```python
from build123d import *

# Parameters (mm, degrees)
CUT_EXTRUDE1_REACH                              = 51.117
CBORE_FOR_M4_SOCKET_HEAD_CAP_SCREW1_D           = 4.5
CBORE_FOR_M4_SOCKET_HEAD_CAP_SCREW1_CBORE_D     = 8
CBORE_FOR_M4_SOCKET_HEAD_CAP_SCREW1_CBORE_DEPTH = 4.4
CHAMFER1_SIZE                                   = 1
CHAMFER2_SIZE                                   = 0.3


with BuildPart() as part:
    # Sketch1 → Revolve1 (revolve)
    with BuildSketch(Plane.XY, mode=Mode.PRIVATE) as revolve1_sk:
        Polygon((-21, 0), (-21, 16.5), (0, 16.5), (0, 27.5), (9, 27.5), (9, 16.5), (28, 16.5), (28, 0), align=None)
    revolve(revolve1_sk.sketch.rotate(Axis((-30.202765387, 0, 0), (1, 0, 0)), 90), axis=Axis((-30.202765387, 0, 0), (1, 0, 0)))

    # Sketch2 → Cut-Revolve1 (revolve, cut)
    with BuildSketch(Plane.XY, mode=Mode.PRIVATE) as cut_revolve1_sk:
        Polygon((-21, 0), (-21, 13), (-5, 13), (-5, 11), (20, 11), (20, 13), (28, 13), (28, 0), align=None)
    revolve(cut_revolve1_sk.sketch.rotate(Axis((-25.491403617, 0, 0), (1, 0, 0)), 90), axis=Axis((-25.491403617, 0, 0), (1, 0, 0)), mode=Mode.SUBTRACT)

    # Sketch5 → Cut-Extrude1 (cut, up to next)
    with BuildSketch(Plane(origin=(9, 0, 0), x_dir=(0, 0, -1), z_dir=(1, 0, 0)), mode=Mode.PRIVATE) as cut_extrude1_sk1:
        with BuildLine():
            Line((18.5, 20.346989949), (18.5, -20.346989949))
            ThreePointArc((18.5, -20.346989949), (27.5, 0), (18.5, 20.346989949))
        make_face()
    cut_extrude1_tool1 = extrude(cut_extrude1_sk1.sketch, amount=-CUT_EXTRUDE1_REACH, mode=Mode.PRIVATE) & part.part
    add(cut_extrude1_tool1.solids().sort_by_distance((9, 0, -22.155812))[0], mode=Mode.SUBTRACT)

    # CBORE for M4 Socket Head Cap Screw1 (through all)
    with Locations(Plane(origin=(9, 0, 0), x_dir=(0, 0, -1), z_dir=(1, 0, 0))):
        with Locations((-13.25, 18), (13.25, 18), (13.25, -18), (-13.25, -18)):
            CounterBoreHole(CBORE_FOR_M4_SOCKET_HEAD_CAP_SCREW1_D / 2, CBORE_FOR_M4_SOCKET_HEAD_CAP_SCREW1_CBORE_D / 2, CBORE_FOR_M4_SOCKET_HEAD_CAP_SCREW1_CBORE_DEPTH)

    # Chamfer1
    chamfer1_edges = [part.edges().sort_by_distance(p)[0] for p in [
        (-21, 0, -16.5),
    ]]
    chamfer(chamfer1_edges, length=CHAMFER1_SIZE)

    # Chamfer2
    chamfer2_edges = [part.edges().sort_by_distance(p)[0] for p in [
        (28, 0, -16.5),
    ]]
    chamfer(chamfer2_edges, length=CHAMFER2_SIZE)


solid = part.part
```
Geometry: final body of the model. Coordinates: model frame, mm. A direction names the side the tool comes from. Round coordinates to 2 decimals unless told otherwise and drop trailing zeros. Write each loop counter-clockwise with the first axis right and the second up, starting at its lowest first coordinate (ties: lowest second). Pieces come first, ordered by that corner, then holes. Notation, with made-up numbers: M 81,-12.5 L 111,-12.5 A22 cw 111,2.5 Z; hole C -27.5,62 d9. An arc over 180 degrees is marked long. Answer in a Markdown table with one row per item. Add a question column.
(1) Ray query, L1, parallel to Y at x = 2.95, z = 13.25; L2, parallel to Y at x = 3, z = -12; L3, parallel to X at y = 19.5, z = -16. Return the intervals inside material, ascending.
(2) Contact query for flat-ended pins moving along their axis: pin 1 (12 mm diameter, centred on x = 17.5, z = 12.5, fed in from -Y); pin 2 (5 mm diameter, centred on x = 15.5, y = 10, fed in from +Z); pin 3 (12 mm diameter, centred on x = -7.5, z = -1, fed in from -Y). Output: stop coordinate, or through.
(3) Cut plane C-C, the plane y = 0. Return the cut outline in (x, z), then the cut area to 3 significant figures.
(4) Draft query along Z for faces 1 (the face through (28, -13.3, -0.1)), 2 (the face through (24.056, 7.91, -10.316)), 3 (the face through (18.481, -4.956, 15.738)). Return one class per face: pulls with the +Z half, pulls with the -Z half, needs draft (parallel to the pull), parting line crosses it, or undercut.
(5) Reachability of faces 4 (the face through (-21, 13, -3)), 5 (the face through (4.6, -20, -15)), 6 (the face through (-5, -3, -11)) from +Z, -Z, +X, -X, +Y, -Y: full face, straight path, thin tool, end or side. Return the list, or none.
(6) Cut plane B-B, the plane x = 2.5. Return the cut outline in (y, z), then the cut area to 3 significant figures.
(7) Cut plane A-A, the plane z = 0. Return the cut outline in (x, y), then the cut area to 3 significant figures.
(8) Cut plane D-D, the plane y = -18. Return the cut outline in (x, z), then the cut area to 3 significant figures.
Established:
| question | item | result |
|---|---|---|
| 1 | L1 | -24.1 to -20.25, -15.75 to 15.75, 20.25 to 24.1 |
| 1 | L2 | -24.74 to -19.87, -16.13 to 16.13, 19.87 to 24.74 |
| 1 | L3 | 0 to 4.6 |
| 2 | pin 1 | y = -15.17 |
| 2 | pin 2 | z = 14.7 |
| 2 | pin 3 | y = -16.5 |
| 3 | outline | M -21,-15.5 L -20,-16.5 L 0,-16.5 L 0,-18.5 L 9,-18.5 L 9,-16.5 L 27.7,-16.5 L 28,-16.2 L 28,-13 L 20,-13 L 20,-11 L -5,-11 L -5,-13 L -21,-13 Z; M -21,13 L -5,13 L -5,11 L 20,11 L 20,13 L 28,13 L 28,16.2 L 27.7,16.5 L 9,16.5 L 9,27.5 L 0,27.5 L 0,16.5 L -20,16.5 L -21,15.5 Z |
| 3 | area | 559 mm² |
| 4 | face 1 | needs draft |
| 4 | face 2 | undercut |
| 4 | face 3 | parting line crosses it |
| 5 | face 4 | +Z, -Z, -X, +Y, -Y |
| 5 | face 5 | +X |
| 5 | face 6 | -X |
| 6 | outline | M -20.35,-18.5 L 20.35,-18.5 A27.5 ccw long Z; hole C -18,-13.25 d4.5; hole C -18,13.25 d4.5; hole C 0,0 d22; hole C 18,-13.25 d4.5; hole C 18,13.25 d4.5 |
| 6 | area | 1,680 mm² |
| 7 | outline | M -21,-15.5 L -20,-16.5 L 0,-16.5 L 0,-27.5 L 9,-27.5 L 9,-16.5 L 27.7,-16.5 L 28,-16.2 L 28,-13 L 20,-13 L 20,-11 L -5,-11 L -5,-13 L -21,-13 Z; M -21,13 L -5,13 L -5,11 L 20,11 L 20,13 L 28,13 L 28,16.2 L 27.7,16.5 L 9,16.5 L 9,27.5 L 0,27.5 L 0,16.5 L -20,16.5 L -21,15.5 Z |
| 7 | area | 640 mm² |
| 8 | outline | M 0,-18.5 L 9,-18.5 L 9,-17.25 L 4.6,-17.25 L 4.6,-15.5 L 0,-15.5 Z; M 0,-11 L 4.6,-11 L 4.6,-9.25 L 9,-9.25 L 9,9.25 L 4.6,9.25 L 4.6,11 L 0,11 Z; M 0,15.5 L 4.6,15.5 L 4.6,17.25 L 9,17.25 L 9,20.79 L 0,20.79 Z |
| 8 | area | 242 mm² |
